For this review, take the finished solid that the model builds, in its own axes (mm). A direction names the side the tool comes from. Round coordinates to 2 decimals unless told otherwise and drop trailing zeros. Order: outer loops, then holes, each group sorted by start corner. A loop starts at its lowest first (then second) coordinate and runs counter-clockwise, first axis right, second up. Notation, with made-up numbers: (52, -14) -> (75, -14) arc R11 ccw to (75, 2) -> close; hole circle Ø5 at (87.25, 75.25). An arc over 180 degrees is marked (long way). Use a Markdown table: item, result. Add a question column.
1) Consider section A-A (y = -0.75). State the section outline as (x, z) points, plus the area to 3 significant figures.
2) Wall thickness on line 1 along Y through (x, z) = (-10, -7); line 2 along X through (y, z) = (-5, -16); line 3 along X through (y, z) = (-1, 2.5): over which ranges is each line inside the solid? List them lowest first. Write a range as [from, to].
3) Draft analysis for pull direction Z (two halves, no side actions). For faces 1 (the face through (-15.343, -0.057, -8.905)), 2 (the face through (-18.91, -0.06, 4.32)), 3 (the face through (7.8, -7.112, 4.66)), 4 (the face through (-4.1, -5.7, 20.97)), state which applies: pulls with the +Z half, pulls with the -Z half, needs draft (parallel to the pull), parting line crosses it, or undercut.
4) Clearance check with flat-ended pins moving along their axes: P1, Ø1.5, axis at y = -5, z = 4, coming from the -X side; P2, Ø8, axis at y = 3.5, z = 5, coming from the +X side; P3, Ø2, axis at y = -0.5, z = 11.5, coming from the -X side. State where each tip first meets the part, or that it passes through.
5) Machinability: for faces 5 (the face through (-14.837, -5.698, -9.42)), 6 (the face through (8.056, -6.726, 5.578)), 7 (the face through (8.619, -0.057, -15.194)), which of the approach directions +Z, -Z, +X, -X, +Y, -Y give a long, thin tool a straight path to every point of the face, cutting with its end or side? Answer none if there is none.
6) Consider section B-B (y = -5). State the section outline as (x, z) points, plus the area to 3 significant figures.
```python
from build123d import *

# Parameters (mm, degrees)
F2_DEPTH = 6.35
F4_F1_R  = 2.286
F4_F2_R  = 2.286
F9_DEPTH = 0.762
F7_DEPTH = 0.762


with BuildPart() as f2:
    # F1 (on face) → F2 (new body, symmetric)
    with BuildSketch(Plane.XZ):
        Polygon((-22.4694542891, -22.4946287922), (0, -10.6504899906), (0, 35.9793268616), (-7.7678262384, 11.7962568429), (-33.1678262384, 11.7962568429), (-10.6731974462, 0), align=None)
    extrude(amount=F2_DEPTH, both=True)

    # F3: F2 across plane


with BuildPart() as f2_1:
    add(f2.part)
    add(f2.part.mirror(Plane.YZ))

    # F4: fillet of radius 2.286 on 26 edges, made by hand

    # F4_f1
    f4_f1_edges = [f2_1.edges().sort_by_distance(p)[0] for p in [
        (7.7678262384, 0, 11.7962568429),
        (10.6731974462, 0, 0),
        (0, 0, -10.6504899906),
        (-10.6731974462, 0, 0),
        (-7.7678262384, 0, 11.7962568429),
    ]]
    fillet(f4_f1_edges, radius=F4_F1_R)

    # F4_f2
    f4_f2_edges = [f2_1.edges().sort_by_distance(p)[0] for p in [
        (-11.7677133906, -6.35, -16.8535080516),
        (11.7677133906, -6.35, -16.8535080516),
        (17.1021574256, -6.35, -12.2595726917),
        (22.932770138, -6.35, 6.4289599794),
        (21.3012015954, -6.35, 11.7962568429),
        (3.6290503253, -6.35, 24.6812396715),
        (-3.6290503253, -6.35, 24.6812396715),
        (-21.3012015954, -6.35, 11.7962568429),
        (-22.932770138, -6.35, 6.4289599794),
        (-17.1021574256, -6.35, -12.2595726917),
        (0, 0, 35.9793268616),
        (3.6290503253, 6.35, 24.6812396715),
        (21.3012015954, 6.35, 11.7962568429),
        (33.1678262384, 0, 11.7962568429),
        (17.1021574256, 6.35, -12.2595726917),
        (22.4694542891, 0, -22.4946287922),
        (-11.7677133906, 6.35, -16.8535080516),
        (-22.4694542891, 0, -22.4946287922),
        (-22.932770138, 6.35, 6.4289599794),
        (-33.1678262384, 0, 11.7962568429),
        (-21.3012015954, 6.35, 11.7962568429),
        (-8.0877949674, 6.35, 12.2351038213),
        (-11.5771185545, 6.35, -0.2820132537),
        (0, 6.35, -10.948638197),
        (11.5771185545, 6.35, -0.2820132537),
        (8.0877949674, 6.35, 12.2351038213),
        (-11.5771185545, -6.35, -0.2820132537),
        (-8.0877949674, -6.35, 12.2351038213),
        (8.0877949674, -6.35, 12.2351038213),
        (11.5771185545, -6.35, -0.2820132537),
        (0, -6.35, -10.948638197),
    ]]
    fillet(f4_f2_edges, radius=F4_F2_R)

    # F8 (on face) → F9 (join)
    with BuildSketch(Plane.XZ.offset(6.35)):
        Polygon((-4.8077497631, 6.9738719612), (-4.8833619803, 6.9888005964), (-5.6563438848, 6.9888005964), (-6.2521840446, 6.6184131429), (-6.1394576915, 5.9903655201), (-5.3503718227, 5.4911477491), (-4.8953713849, 5.0424882211), (-4.8953713849, 4.3044914491), (-5.5958377197, 3.9264927618), (-6.1300005764, 3.9264927618), (-6.4605637453, 4.0734503418), (-6.6418400966, 3.6255908199), (-6.0233678669, 3.4443144687), (-5.4048956372, 3.4976312891), (-4.8717297614, 3.7642139941), (-4.5411670581, 4.180083517), (-4.583820235, 4.7665657476), (-4.8717297614, 5.3743747994), (-5.3089256398, 5.7795806788), (-5.7567846961, 6.078153383), (-5.9060710482, 6.4300429076), (-5.5541819893, 6.6433092579), (-5.223619286, 6.6433092579), (-4.9463729374, 6.7606056109), align=None)
    extrude(amount=F9_DEPTH)

    # F6 (on face) → F7 (join)
    with BuildSketch(Plane.XZ.offset(6.35)):
        Polygon((-2.7460011188, 6.3680754974), (-2.852873411, 6.4385421574), (-2.852873411, 5.140052177), (-2.6468993165, 3.9846990258), (-1.7563264119, 3.4034063574), (-0.6719225785, 3.1792041846), (-0.124490587, 3.912220709), (-0.1830757828, 5.1394319162), (-0.1522420207, 6.2248986214), (-0.5077649839, 6.2937401235), (-0.8040870307, 4.9930457026), (-0.7814072305, 3.8545557763), (-1.6878197202, 3.9909644984), (-2.3294347338, 4.5027183369), (-2.3874049075, 5.5876043625), (-2.337427577, 6.3529536128), (-2.7812926564, 6.314471364), align=None)
        Polygon((1.3429354876, 5.8594592847), (1.2765517458, 5.9258458205), (1.2765517458, 2.9113423079), (1.7961976118, 2.7786572464), (1.7949150642, 4.5979730785), (3.0550148804, 5.0231530331), align=None)
        Polygon((2.2798031569, 5.1395706832), (1.7628639471, 4.9090404063), (1.8159369938, 5.3025046363), align=None, mode=Mode.SUBTRACT)
        Polygon((5.8496114798, 6.0712443665), (4.3209996074, 6.0321558267), (4.3209996074, 4.947821144), (4.3456433341, 2.8858925216), (5.8767511191, 2.904191992), (5.8767511191, 3.2648150809), (4.8615592532, 3.2685473561), (4.8615592532, 4.235221073), (5.6510670111, 4.220648203), (5.6144981645, 4.6745948493), (4.8782676458, 4.666226916), (4.8519740812, 5.6559145451), (5.933160428, 5.6408806704), align=None)
        Polygon((7.0347818546, 6.3396086916), (7.0347818546, 2.9729763046), (7.4759777635, 3.9922273718), (9.0028224513, 2.937797457), (7.6884618029, 4.3934863061), (9.0492879972, 4.8372442834), align=None)
        Polygon((8.0597589084, 4.9393000391), (7.7467951924, 4.8372442834), (7.6166405343, 4.8372442834), (7.6166405343, 5.243926309), align=None, mode=Mode.SUBTRACT)
    extrude(amount=F7_DEPTH)


solid = f2_1.part
```
Results list:
| question | item | result |
|---|---|---|
| 1 | outline | (-24.95, 7.49) -> (-12.7, 1.06) arc R2.29 cw to (-11.73, -2.02) -> (-19.05, -15.98) arc R2.29 ccw to (-15.96, -19.07) -> (-1.07, -11.21) arc R2.29 cw to (1.07, -11.21) -> (15.96, -19.07) arc R2.29 ccw to (19.05, -15.98) -> (11.73, -2.02) arc R2.29 cw to (12.7, 1.06) -> (24.95, 7.49) arc R2.29 ccw to (23.89, 11.8) -> (9.43, 11.8) arc R2.29 cw to (7.26, 13.38) -> (2.18, 29.2) arc R2.29 ccw to (-2.18, 29.2) -> (-7.26, 13.38) arc R2.29 cw to (-9.43, 11.8) -> (-23.89, 11.8) arc R2.29 ccw to start |
| 1 | area | 1,130 mm2 |
| 2 | line 1 | [-6.35, 6.35] |
| 2 | line 2 | [-18.84, -10.58], [10.58, 18.84] |
| 2 | line 3 | [-15.44, 15.44] |
| 3 | face 1 | undercut |
| 3 | face 2 | undercut |
| 3 | face 3 | needs draft |
| 3 | face 4 | pulls with the +Z half |
| 4 | P1 | x = -19.42 |
| 4 | P2 | x = 26.11 |
| 4 | P3 | x = -25.95 |
| 5 | face 5 | -X, -Y |
| 5 | face 6 | +Z, +X, -Y |
| 5 | face 7 | -Z, +Y, -Y |
| 6 | outline | (-24.85, 7.66) -> (-12.6, 1.24) arc R2.49 cw to (-11.56, -2.12) -> (-18.88, -16.07) arc R2.09 ccw to (-16.06, -18.89) -> (-1.16, -11.04) arc R2.49 cw to (1.16, -11.04) -> (16.06, -18.89) arc R2.09 ccw to (18.88, -16.07) -> (11.56, -2.12) arc R2.49 cw to (12.6, 1.24) -> (24.85, 7.66) arc R2.09 ccw to (23.89, 11.6) -> (9.43, 11.6) arc R2.49 cw to (7.07, 13.32) -> (1.99, 29.14) arc R2.09 ccw to (-1.99, 29.14) -> (-7.07, 13.32) arc R2.49 cw to (-9.43, 11.6) -> (-23.89, 11.6) arc R2.09 ccw to start |
| 6 | area | 1,090 mm2 |
